Geometry check sheet. Reference: the model listing, model coordinates, mm. Face numbers are marked on the shaded views. A direction names the side the tool comes from. Round coordinates to 2 decimals unless told otherwise and drop trailing zeros. Loops run counter-clockwise (first coordinate to the right, second up) from the corner with the lowest first, then second, coordinate; pieces in that order, holes last. Notation, with made-up numbers: M 74.5,23 L 94.5,23 A23 ccw 94.5,42 Z; hole C 38.25,-14.5 d6. An arc over 180 degrees is marked long. Use one line per item in the form item = value. Start each with the question number.
1. Cross-section at D-D (z = -8). Record the boundary of the cut face in (x, y).
2. Cross-section at B-B (z = 0). Record the boundary of the cut face in (x, y).
3. Cross-section at C-C (x = 8.5). Record the boundary of the cut face in (y, z), then the cut area to 3 significant figures.
4. Cross-section at A-A (y = -7.25). State how many separate pieces and enclosed holes the cut face has, then the cut area to 3 significant figures.
5. Set-up check for the marked faces 1, 2 and 3: record each of +Z, -Z, +X, -X, +Y, -Y from which the full face is reachable in a straight line by a thin tool's end or side.
6. Material ranges on line 1 (X direction, y = -8, z = -2.5); line 2 (X direction, y = -2, z = -13); line 3 (X direction, y = -2, z = -15), recorded low to high.
7. Go/stop test with flat-tipped pins: pin 1 (2 mm diameter, centred on x = 19, z = 4, fed in from -Y); pin 2 (4 mm diameter, centred on x = -14.85, z = -14.85, fed in from -Y); pin 3 (2.5 mm diameter, centred on x = -22, y = -10.5, fed in from +Z); pin 4 (2 mm diameter, centred on y = -10.5, z = -17, fed in from +X). Record where each tip stops, or that it passes through.
8. Draft check along X on the marked faces 4, 5, 6 and 7. Enter one of: pulls with the +X half, pulls with the -X half, needs draft (parallel to the pull), parting line crosses it, or undercut.
```python
from build123d import *
from build123d.topology import SkipClean

# Parameters (mm, degrees)
SKETCH4_R           = 26
SKETCH4_R_2         = 2.1
SKETCH4_R_3         = 1.55
BOSS_EXTRUDE1_DEPTH = 4
SKETCH5_R           = 1.55
SKETCH5_R_2         = 2.1
BOSS_EXTRUDE2_DEPTH = 10
CUT_EXTRUDE1_START  = -8
CUT_EXTRUDE1_DEPTH  = 8
FILLET1_R           = 1


with BuildPart() as part:
    # Sketch4 → Boss-Extrude1 (new body)
    with BuildSketch(Plane(origin=(0, 0, 3), x_dir=(1, 0, 0), z_dir=(0, -1, 0))):
        with Locations(Location((0, -3, 0), (0, 0, 270))):
            Circle(SKETCH4_R)
        with Locations(Location((0, 18, 0), (0, 0, 270))):
            Circle(SKETCH4_R_2, mode=Mode.SUBTRACT)
        with Locations(Location((7.653668647, 15.47759065, 0), (0, 0, 270))):
            Circle(SKETCH4_R_3, mode=Mode.SUBTRACT)
        with Locations(Location((14.849242405, 11.849242405, 0), (0, 0, 270))):
            Circle(SKETCH4_R_2, mode=Mode.SUBTRACT)
        with Locations(Location((18.47759065, 4.653668647, 0), (0, 0, 270))):
            Circle(SKETCH4_R_3, mode=Mode.SUBTRACT)
        with Locations(Location((21, -3, 0), (0, 0, 270))):
            Circle(SKETCH4_R_2, mode=Mode.SUBTRACT)
        with Locations(Location((18.47759065, -10.653668647, 0), (0, 0, 270))):
            Circle(SKETCH4_R_3, mode=Mode.SUBTRACT)
        with Locations(Location((14.849242405, -17.849242405, 0), (0, 0, 270))):
            Circle(SKETCH4_R_2, mode=Mode.SUBTRACT)
        with Locations(Location((7.653668647, -21.47759065, 0), (0, 0, 270))):
            Circle(SKETCH4_R_3, mode=Mode.SUBTRACT)
        with Locations(Location((0, -24, 0), (0, 0, 270))):
            Circle(SKETCH4_R_2, mode=Mode.SUBTRACT)
        with Locations(Location((-7.653668647, -21.47759065, 0), (0, 0, 270))):
            Circle(SKETCH4_R_3, mode=Mode.SUBTRACT)
        with Locations(Location((-14.849242405, -17.849242405, 0), (0, 0, 270))):
            Circle(SKETCH4_R_2, mode=Mode.SUBTRACT)
        with Locations(Location((-18.47759065, -10.653668647, 0), (0, 0, 270))):
            Circle(SKETCH4_R_3, mode=Mode.SUBTRACT)
        with Locations(Location((-21, -3, 0), (0, 0, 270))):
            Circle(SKETCH4_R_2, mode=Mode.SUBTRACT)
        with Locations(Location((-18.47759065, 4.653668647, 0), (0, 0, 270))):
            Circle(SKETCH4_R_3, mode=Mode.SUBTRACT)
        with Locations(Location((-14.849242405, 11.849242405, 0), (0, 0, 270))):
            Circle(SKETCH4_R_2, mode=Mode.SUBTRACT)
        with Locations(Location((-7.653668647, 15.47759065, 0), (0, 0, 270))):
            Circle(SKETCH4_R_3, mode=Mode.SUBTRACT)
    extrude(amount=BOSS_EXTRUDE1_DEPTH)

    # Sketch5 → Boss-Extrude2 (add)
    # profile 1 of 2: a face of its own
    with SkipClean():  # the faces are left unmerged after this step: merging them gives an invalid solid
        with BuildSketch(Plane.XZ.offset(4)):
            with BuildLine():
                Line((-12.5, 22.79802623), (-12.5, -22.79802623))
                ThreePointArc((-12.5, -22.79802623), (-26, 0), (-12.5, 22.79802623))
            make_face()
            with Locations(Location((-18.47759065, 7.653668647, 0), (0, 0, 270))):
                Circle(SKETCH5_R, mode=Mode.SUBTRACT)
            with Locations(Location((-18.47759065, -7.653668647, 0), (0, 0, 270))):
                Circle(SKETCH5_R, mode=Mode.SUBTRACT)
            with Locations(Location((-14.849242405, -14.849242405, 0), (0, 0, 270))):
                Circle(SKETCH5_R_2, mode=Mode.SUBTRACT)
            with Locations(Location((-21, 0, 0), (0, 0, 270))):
                Circle(SKETCH5_R_2, mode=Mode.SUBTRACT)
            with Locations(Location((-14.849242405, 14.849242405, 0), (0, 0, 270))):
                Circle(SKETCH5_R_2, mode=Mode.SUBTRACT)
        # profile 2 of 2: a face of its own
        with BuildSketch(Plane.XZ.offset(4)):
            with BuildLine():
                Line((12.5, -22.79802623), (12.5, 22.79802623))
                ThreePointArc((12.5, 22.79802623), (26, 0), (12.5, -22.79802623))
            make_face()
            with Locations(Location((18.47759065, -7.653668647, 0), (0, 0, 270))):
                Circle(SKETCH5_R, mode=Mode.SUBTRACT)
            with Locations(Location((18.47759065, 7.653668647, 0), (0, 0, 270))):
                Circle(SKETCH5_R, mode=Mode.SUBTRACT)
            with Locations(Location((14.849242405, 14.849242405, 0), (0, 0, 270))):
                Circle(SKETCH5_R_2, mode=Mode.SUBTRACT)
            with Locations(Location((21, 0, 0), (0, 0, 270))):
                Circle(SKETCH5_R_2, mode=Mode.SUBTRACT)
            with Locations(Location((14.849242405, -14.849242405, 0), (0, 0, 270))):
                Circle(SKETCH5_R_2, mode=Mode.SUBTRACT)
        extrude(amount=BOSS_EXTRUDE2_DEPTH)

    # Sketch6 → Cut-Extrude1 (cut)
    with SkipClean():  # the faces are left unmerged after this step: merging them gives an invalid solid
        with BuildSketch(Plane.XZ.offset(14).offset(CUT_EXTRUDE1_START)):
            with BuildLine():
                Line((21, 4.75), (25.562423594, 4.75))
                ThreePointArc((25.562423594, 4.75), (26, 0), (25.562423594, -4.75))
                Line((25.562423594, -4.75), (21, -4.75))
                ThreePointArc((21, -4.75), (16.25, 0), (21, 4.75))
            make_face()
            with BuildLine():
                Line((-21, -4.75), (-25.562423594, -4.75))
                ThreePointArc((-25.562423594, -4.75), (-26, 0), (-25.562423594, 4.75))
                Line((-25.562423594, 4.75), (-21, 4.75))
                ThreePointArc((-21, 4.75), (-16.25, 0), (-21, -4.75))
            make_face()
        extrude(amount=CUT_EXTRUDE1_DEPTH, mode=Mode.SUBTRACT)

    # Fillet1
    fillet1_edges = [part.edges().sort_by_distance(p)[0] for p in [
        (-25.562423594, -10, -4.75),
        (-25.562423594, -10, 4.75),
        (25.562423594, -10, 4.75),
        (25.562423594, -10, -4.75),
        (-12.5, -9, 22.79802623),
        (-12.5, -9, -22.79802623),
        (12.5, -9, -22.79802623),
        (12.5, -9, 22.79802623),
    ]]
    fillet(fillet1_edges, radius=FILLET1_R)


solid = part.part
```
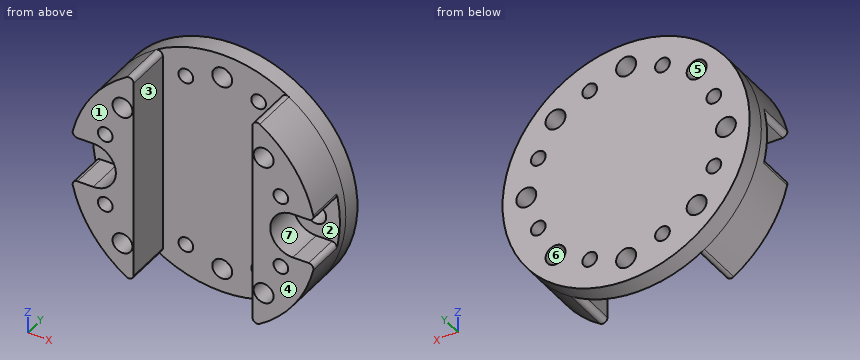
Reported:
q1.outline = M -24.74,-14 L -19.99,-14 L -19.99,0 L -24.74,0 Z; M -16.97,-14 L -12.5,-14 L -12.5,-4 L 12.5,-4 L 12.5,-14 L 16.97,-14 L 16.97,0 L -16.97,0 Z; M 19.99,-14 L 24.74,-14 L 24.74,0 L 19.99,0 Z
q2.outline = M -26,-6 L -23.1,-6 L -23.1,0 L -26,0 Z; M -18.9,-6 L -16.25,-6 L -16.25,-14 L -12.5,-14 L -12.5,-4 L 12.5,-4 L 12.5,-14 L 16.25,-14 L 16.25,-6 L 18.9,-6 L 18.9,0 L -18.9,0 Z; M 23.1,-6 L 26,-6 L 26,0 L 23.1,0 Z
q3.outline = M -4,-24.57 L 0,-24.57 L 0,-19.78 L -4,-19.78 Z; M -4,-17.18 L 0,-17.18 L 0,17.18 L -4,17.18 Z; M -4,19.78 L 0,19.78 L 0,24.57 L -4,24.57 Z
q3.area = 176 mm²
q4.separate_pieces = 2
q4.enclosed_holes = 8
q4.area = 623 mm²
q5.face_1 = +Z, -Z, +X, -X, -Y
q5.face_2 = +X, -Y
q5.face_3 = +Z, -Z, -Y
q6.line_1 = -16.96 to -12.5, 12.5 to 16.96
q6.line_2 = -22.52 to -15.84, -13.85 to 13.85, 15.84 to 22.52
q6.line_3 = -21.24 to -16.94, -12.75 to 12.75, 16.94 to 21.24
q7.pin_1 = -14
q7.pin_2 = through
q7.pin_3 = 15.67
q7.pin_4 = 20.49
q8.face_4 = needs draft
q8.face_5 = undercut
q8.face_6 = undercut
q8.face_7 = pulls with the +X half
